from build123d import *

# Parameters (mm, degrees)
SKETCH_1_R               = 15
EXTRUDE_1_DEPTH          = 20
SKETCH_2_R               = 5
EXTRUDE_2_DEPTH          = 5
SKETCH_3_W               = 2
SKETCH_3_H               = 2
CUT_EXTRUDE_1_DEPTH      = 33.787192622
PATTERN_CIRCULAR_1_COUNT = 12
SKETCH_4_R               = 3
CUT_EXTRUDE_2_DEPTH      = 12


with BuildPart() as part:
    # Sketch 1 → Extrude 1 (new body)
    with BuildSketch(Plane(origin=(0, 0, 0), x_dir=(1, 0, 0), z_dir=(0, 1, 0))):
        with Locations(Location((0, 0, 0), (0, 0, 270))):
            Circle(SKETCH_1_R)
    extrude(amount=EXTRUDE_1_DEPTH)

    # Sketch 2 → Extrude 2 (add)
    with BuildSketch(Plane(origin=(0, 20, 0), x_dir=(1, 0, 0), z_dir=(0, 1, 0))):
        with Locations(Location((0, 0, 0), (0, 0, 270))):
            Circle(SKETCH_2_R)
    extrude(amount=EXTRUDE_2_DEPTH)

    # Sketch 3 → Cut-Extrude 1 (cut, through all)
    with BuildSketch(Plane(origin=(0, 0, 0), x_dir=(1, 0, 0), z_dir=(0, 1, 0))):
        with Locations((15, 0)):
            Rectangle(SKETCH_3_W, SKETCH_3_H)
    cut_extrude_1 = extrude(amount=CUT_EXTRUDE_1_DEPTH, mode=Mode.SUBTRACT)

    # Pattern Circular 1: Cut-Extrude 1 ×12 about axis
    pattern_circular_1_axis = Axis((0, 0, 0), (0, 1, 0))
    for i in range(1, PATTERN_CIRCULAR_1_COUNT):
        add(cut_extrude_1.rotate(pattern_circular_1_axis, i * 360 / PATTERN_CIRCULAR_1_COUNT), mode=Mode.SUBTRACT)

    # Sketch 4 → Cut-Extrude 2 (cut)
    with BuildSketch(Plane(origin=(0, 0, 0), x_dir=(1, 0, 0), z_dir=(0, 1, 0))):
        with Locations(Location((0, 0, 0), (0, 0, 270))):
            Circle(SKETCH_4_R)
    extrude(amount=CUT_EXTRUDE_2_DEPTH, mode=Mode.SUBTRACT)


solid = part.part
Geometry check sheet. Reference: the model listing, model coordinates, mm. A direction names the side the tool comes from. Round coordinates to 2 decimals unless told otherwise and drop trailing zeros. Write each loop counter-clockwise with the first axis right and the second up, starting at its lowest first coordinate (ties: lowest second). Pieces come first, ordered by that corner, then holes. Notation, with made-up numbers: (59, -22) -> (73, -22) arc R21 ccw to (73, 7) -> close; hole circle Ø8 at (16.25, -36.5). An arc over 180 degrees is marked (long way). One line per item, written item: value. Start each with the question number.
(1) Go/stop test with flat-tipped pins: pin 1 Ø2 at (y, z) = (21.5, -1.5) entering from +X; pin 2 Ø3 at (y, z) = (18, -6.5) entering from +X; pin 3 Ø0.6 at (x, y) = (-0.5, 5.5) entering from -Z. Record where each tip stops, or that it passes through.
(2) Draft check along Z on faces 1 (the flat face through (-13.037, 9.86, -6.372)), 2 (the flat face through (13.037, 9.86, 6.372)), 3 (the flat face through (-7.01, 9.86, 12.12)). Enter one of: +Z half, -Z half, draft (parallel to the pull), parting line (faces both ways), or undercut.
(3) Scan lines: line 1 (X direction, y = 3, z = 0); line 2 (Y direction, x = 7, z = -3); line 3 (X direction, y = 20.25, z = -2.5). Record each from-to range of solid material in increasing order. Write a range as [from, to].
(4) Cross-section at A-A, the plane z = 0. Record the cut outline in (x, y), and give its area (3 significant figures).
(5) Access from +Z, -Z, +X, -X, +Y, -Y to the whole of each face (thin tool, end or side, straight path). Record for faces 4 (the flat face through (-13.037, 9.86, 6.372)), 5 (the flat face through (-1, 9.9, -14.5)), 6 (the flat face through (14.5, 9.9, -1)).
(6) Cross-section at C-C, the plane z = 8.75. Record the cut outline in (x, y), and give its area (3 significant figures).
(7) Cross-section at B-B, the plane y = 20.75. Record the cut outline in (x, z).
Answer:
1. pin 1: x = 4.97
1. pin 2: x = 14.14
1. pin 3: z = -14
2. face 1: -Z half
2. face 2: +Z half
2. face 3: undercut
3. line 1: [-14, -3], [3, 14]
3. line 2: [0, 20]
3. line 3: [-4.33, 4.33]
4. outline: (-14, 0) -> (-3, 0) -> (-3, 12) -> (3, 12) -> (3, 0) -> (14, 0) -> (14, 20) -> (5, 20) -> (5, 25) -> (-5, 25) -> (-5, 20) -> (-14, 20) -> close
4. area: 538 mm²
5. face 4: +Z, +Y, -Y
5. face 5: -Z, +Y, -Y
5. face 6: +X, +Y, -Y
6. outline: (-12.18, 0) -> (12.18, 0) -> (12.18, 20) -> (-12.18, 20) -> close
6. area: 487 mm²
7. outline: circle Ø10 at (0, 0)
